Read the model definition and answer for the solid it produces. Units are mm, in the model's axes. A direction names the side the tool comes from. Coordinates: 2 decimals unless noted, no trailing zeros. Write each loop counter-clockwise with the first axis right and the second up, starting at its lowest first coordinate (ties: lowest second). Pieces come first, ordered by that corner, then holes.
Item 1: A tool of negligible diameter and unlimited length cuts with its end or side. For faces 5 (the face through (11.17, -2.3, -9.04)), 6 (the face through (-9.535, -2, -1)), 7 (the face through (-2, -3.048, -11)), 8 (the face through (-1, -2, -18.459)), from which of +Z, -Z, +X, -X, +Y, -Y can it reach the whole face along a straight path? Write none if from no direction.
Item 2: Section B-B (z = -13.5) is taken. Give the vertices of the cut face in (x, y).
Item 3: Determine the mould class of faces 1 (the face through (-11, -2, -22.523)), 2 (the face through (15.23, -1.5, -11.13)), 3 (the face through (4.35, -2.3, -8.96)), 4 (the face through (7.329, -0.751, -7.856)) for opening direction X: released by +X, released by -X, zero draft, split by the parting line, or undercut.
Item 4: Straight lines are drawn through the part: probe 1 along Z at (x, y) = (-3.5, -0.75); probe 2 along Y at (x, z) = (10.75, -9.5); probe 3 along Z at (x, y) = (10.25, -1.4). For each, find the intervals that lie inside material, in ascending order.
Item 5: Section A-A (y = -2.5) is taken. Give the vertices of the cut face in (x, z).
Item 6: Section D-D (z = -8.75) is taken. Give the vertices of the cut face in (x, y), then the cut area to 3 significant figures.
Item 7: Each of these flat-tipped pins is pushed along its axis until it touches: P1, Ø1.5, axis at x = -5, y = -2, coming from the +Z side; P2, Ø2.5, axis at x = 9, z = -9, coming from the -Y side; P3, Ø4, axis at x = 7.74, z = -10.97, coming from the +Y side. Where does it stop, or does it pass through?
Item 8: Section C-C (x = -7) is taken. Give the vertices of the cut face in (y, z).
from build123d import *

# Parameters (mm, degrees)
F0_R     = 3.1369
F1_DEPTH = 3.048
F3_DEPTH = 1.524


with BuildPart() as f1:
    # F0 (on Front) → F1 (new body)
    with BuildSketch(Plane.XZ):
        with BuildLine():
            Line((-9.53489, 0.590851), (-12.70989, 0.590851))
            Line((-12.70989, 0.590851), (-12.70989, -22.523149))
            Line((-12.70989, -22.523149), (-9.53489, -22.523149))
            Line((-9.53489, -22.523149), (-9.53489, -18.459149))
            Line((-9.53489, -18.459149), (7.73711, -18.459149))
            ThreePointArc((7.73711, -18.459149), (15.23011, -10.966149), (7.73711, -3.473149))
            Line((7.73711, -3.473149), (-9.53489, -3.473149))
            Line((-9.53489, -3.473149), (-9.53489, 0.590851))
        make_face()
        with Locations((7.73711, -10.966149)):
            Circle(F0_R, mode=Mode.SUBTRACT)
    extrude(amount=F1_DEPTH)

    # F2 (on face) → F3 (cut)
    with BuildSketch(Plane.XZ.offset(3.048)):
        Polygon((5.478697, -7.020747), (3.191085, -10.949291), (5.449498, -14.894693), (9.995523, -14.911551), (12.283135, -10.983007), (10.024722, -7.037605), align=None)
    extrude(amount=-F3_DEPTH, mode=Mode.SUBTRACT)


solid = f1.part
Established:
1. face 5: -Y
1. face 6: +Z, +X, +Y, -Y
1. face 7: +Z, -Z, +X, -X, -Y
1. face 8: -Z, +X, +Y, -Y
2. outline: (-12.71, -3.05) - (4.65, -3.05) - (4.65, -1.52) - (5.89, -1.52) - (5.89, 0) - (-12.71, 0) - close; (9.59, -1.52) - (10.82, -1.52) - (10.82, -3.05) - (14.79, -3.05) - (14.79, 0) - (9.59, 0) - close
3. face 1: zero draft
3. face 2: released by +X
3. face 3: undercut
3. face 4: undercut
4. probe 1: z = -18.46 to -3.47
4. probe 2: y = -1.52 to 0
4. probe 3: z = -18.03 to -12.84, -9.09 to -3.91
5. outline: (-12.71, -22.52) - (-9.53, -22.52) - (-9.53, -18.46) - (7.74, -18.46) arc R7.49 ccw to (7.74, -3.47) - (-9.53, -3.47) - (-9.53, 0.59) - (-12.71, 0.59) - close; hole (3.19, -10.95) - (5.45, -14.89) - (10, -14.91) - (12.28, -10.98) - (10.02, -7.04) - (5.48, -7.02) - close
6. outline: (-12.71, -3.05) - (4.47, -3.05) - (4.47, -1.52) - (5.52, -1.52) - (5.52, 0) - (-12.71, 0) - close; (9.96, -1.52) - (11, -1.52) - (11, -3.05) - (14.89, -3.05) - (14.89, 0) - (9.96, 0) - close
6. area: 67.4 mm2
7. P1: stops at z = -3.47
7. P2: stops at y = -1.52
7. P3: passes through
8. outline: (-3.05, -18.46) - (0, -18.46) - (0, -3.47) - (-3.05, -3.47) - close
